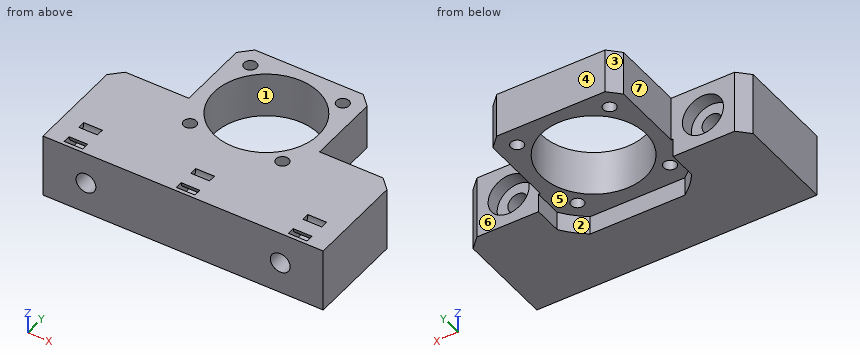
```python
from build123d import *

# Parameters (mm, degrees)
ESQUISSE1_R                                        = 14
ESQUISSE1_R_2                                      = 1.7
BOSS_EXTRU_1_DEPTH                                 = 17
BOSS_EXTRU_2_START                                 = -17
ESQUISSE2_R                                        = 1.7
ESQUISSE2_R_2                                      = 14
BOSS_EXTRU_2_DEPTH                                 = 17
CHAMBRAGE_POUR_VIS_T_TE_RONDE_BOMB_E_M_D           = 5.3
CHAMBRAGE_POUR_VIS_T_TE_RONDE_BOMB_E_M_DEPTH       = 35
CHAMBRAGE_POUR_VIS_T_TE_RONDE_BOMB_E_M_CBORE_D     = 11
CHAMBRAGE_POUR_VIS_T_TE_RONDE_BOMB_E_M_CBORE_DEPTH = 3.7
CHAMBRAGE_POUR_VIS_T_TE_RONDE_BOMB_E_M_TIP         = 1.59228064
ESQUISSE7_W                                        = 5
ESQUISSE7_H                                        = 2
ENL_V_MAT_EXTRU_1_DEPTH                            = 5
ENL_V_MAT_EXTRU_2_DEPTH                            = 5


with BuildPart() as part:
    # Esquisse1 → Boss.-Extru.1 (new body)
    with BuildSketch(Plane.XY):
        with BuildLine():
            Line((12.489995997, 17.5), (-12.489995997, 17.5))
            ThreePointArc((-12.489995997, 17.5), (-15.202795796, 15.202795796), (-17.5, 12.489995997))
            Line((-17.5, 12.489995997), (-17.5, -12.489995997))
            ThreePointArc((-17.5, -12.489995997), (-15.202795796, -15.202795796), (-12.489995997, -17.5))
            Line((-12.489995997, -17.5), (12.489995997, -17.5))
            ThreePointArc((12.489995997, -17.5), (15.202795796, -15.202795796), (17.5, -12.489995997))
            Line((17.5, -12.489995997), (17.5, 12.489995997))
            ThreePointArc((17.5, 12.489995997), (15.202795796, 15.202795796), (12.489995997, 17.5))
        make_face()
        Circle(ESQUISSE1_R, mode=Mode.SUBTRACT)
        with Locations((-12.374368671, -12.374368671)):
            Circle(ESQUISSE1_R_2, mode=Mode.SUBTRACT)
        with Locations((12.374368671, -12.374368671)):
            Circle(ESQUISSE1_R_2, mode=Mode.SUBTRACT)
        with Locations((12.374368671, 12.374368671)):
            Circle(ESQUISSE1_R_2, mode=Mode.SUBTRACT)
        with Locations((-12.374368671, 12.374368671)):
            Circle(ESQUISSE1_R_2, mode=Mode.SUBTRACT)
    extrude(amount=BOSS_EXTRU_1_DEPTH)

    # Esquisse2 → Boss.-Extru.2 (add)
    with BuildSketch(Plane.XY.offset(17).offset(BOSS_EXTRU_2_START)):
        Polygon((-12.489995997, 17.5), (-14.5, 17.5), (-17.5, 14.5), (-17.5, -5), (-34.5, -5), (-37.5, -8), (-37.5, -34.15), (37.5, -34.15), (37.5, -8), (34.5, -5), (17.5, -5), (17.5, 14.5), (14.5, 17.5), align=None)
        with Locations((12.374368671, 12.374368671)):
            Circle(ESQUISSE2_R, mode=Mode.SUBTRACT)
        with Locations((12.374368671, -12.374368671)):
            Circle(ESQUISSE2_R, mode=Mode.SUBTRACT)
        with Locations((-12.374368671, -12.374368671)):
            Circle(ESQUISSE2_R, mode=Mode.SUBTRACT)
        with Locations((-12.374368671, 12.374368671)):
            Circle(ESQUISSE2_R, mode=Mode.SUBTRACT)
        Circle(ESQUISSE2_R_2, mode=Mode.SUBTRACT)
    extrude(amount=BOSS_EXTRU_2_DEPTH)

    # Chambrage pour vis à tête ronde bombée M51
    with Locations(Plane(origin=(0, -5, 0), x_dir=(1, 0, 0), z_dir=(0, 1, 0))):
        with Locations((-26, -8.5), (26, -8.5)):
            CounterBoreHole(CHAMBRAGE_POUR_VIS_T_TE_RONDE_BOMB_E_M_D / 2, CHAMBRAGE_POUR_VIS_T_TE_RONDE_BOMB_E_M_CBORE_D / 2, CHAMBRAGE_POUR_VIS_T_TE_RONDE_BOMB_E_M_CBORE_DEPTH, depth=CHAMBRAGE_POUR_VIS_T_TE_RONDE_BOMB_E_M_DEPTH)
            with Locations((0, 0, -(CHAMBRAGE_POUR_VIS_T_TE_RONDE_BOMB_E_M_DEPTH + CHAMBRAGE_POUR_VIS_T_TE_RONDE_BOMB_E_M_TIP / 2))):  # 118° drill point
                Cone(0, CHAMBRAGE_POUR_VIS_T_TE_RONDE_BOMB_E_M_D / 2, CHAMBRAGE_POUR_VIS_T_TE_RONDE_BOMB_E_M_TIP, mode=Mode.SUBTRACT)

    # Esquisse7 → Enlèvement de matière-Révolution1 (revolve, cut)
    with BuildSketch(Plane.XY.offset(17)):
        with Locations((0, -26.15)):
            Rectangle(ESQUISSE7_W, ESQUISSE7_H)
        with Locations((-30, -26.15)):
            Rectangle(ESQUISSE7_W, ESQUISSE7_H)
        with Locations((30, -26.15)):
            Rectangle(ESQUISSE7_W, ESQUISSE7_H)
    revolve(axis=Axis((-37.5, -29.15, 17), (1, 0, 0)), mode=Mode.SUBTRACT)

    # Esquisse8 → Enlèv. mat.-Extru.1 (cut)
    with BuildSketch(Plane(origin=(0, 0, 0), x_dir=(-1, 0, 0), z_dir=(0, 0, -1))):
        with BuildLine():
            Line((-12.489995997, 17.5), (-14.5, 17.5))
            Line((-14.5, 17.5), (-17.5, 14.5))
            Line((-17.5, 14.5), (-17.5, 12.489995997))
            Line((-17.5, 12.489995997), (-17.5, -12.489995997))
            ThreePointArc((-17.5, -12.489995997), (-15.202795796, -15.202795796), (-12.489995997, -17.5))
            Line((-12.489995997, -17.5), (12.489995997, -17.5))
            ThreePointArc((12.489995997, -17.5), (15.202795796, -15.202795796), (17.5, -12.489995997))
            Line((17.5, -12.489995997), (17.5, 12.489995997))
            Line((17.5, 12.489995997), (17.5, 14.5))
            Line((17.5, 14.5), (14.5, 17.5))
            Line((14.5, 17.5), (12.489995997, 17.5))
            Line((12.489995997, 17.5), (-12.489995997, 17.5))
        make_face()
    extrude(amount=-ENL_V_MAT_EXTRU_1_DEPTH, mode=Mode.SUBTRACT)

    # Esquisse9 → Enlèv. mat.-Extru.2 (cut)
    with BuildSketch(Plane(origin=(0, 0, 0), x_dir=(-1, 0, 0), z_dir=(0, 0, -1))):
        with BuildLine():
            Line((-18, -4.5), (-18, -12.649110641))
            ThreePointArc((-18, -12.649110641), (-15.556349186, -15.556349186), (-12.649110641, -18))
            Line((-12.649110641, -18), (12.649110641, -18))
            ThreePointArc((12.649110641, -18), (15.556349186, -15.556349186), (18, -12.649110641))
            Line((18, -12.649110641), (18, -4.5))
            Line((18, -4.5), (-18, -4.5))
        make_face()
        with BuildLine():
            Line((17.5, -12.489995997), (17.5, -5))
            Line((17.5, -5), (-17.5, -5))
            Line((-17.5, -5), (-17.5, -12.489995997))
            ThreePointArc((-17.5, -12.489995997), (-15.202795796, -15.202795796), (-12.489995997, -17.5))
            Line((-12.489995997, -17.5), (12.489995997, -17.5))
            ThreePointArc((12.489995997, -17.5), (15.202795796, -15.202795796), (17.5, -12.489995997))
        make_face(mode=Mode.SUBTRACT)
    extrude(amount=-ENL_V_MAT_EXTRU_2_DEPTH, mode=Mode.SUBTRACT)


solid = part.part
```
Verification items for the finished model (mm, model axes). Face numbers are marked on the shaded views. A direction names the side the tool comes from. Give positions to 0.01 mm unless a question says otherwise; leave off trailing zeros. Order: outer loops, then holes, each group sorted by start corner. A loop starts at its lowest first (then second) coordinate and runs counter-clockwise, first axis right, second up. Notation, with made-up numbers: M 16,9 L 48,9 A23 ccw 48,30 Z; hole C 15,83 d4. An arc over 180 degrees is marked long. Return JSON: item names as keys, results as strings. Group by question number.
1) Section check D-D on x = 0. Record the cut outline in (y, z).
2) Section check B-B on x = -26. Record the cut outline in (y, z).
3) Mould release check, pull along X, two halves, no side actions. Record for the marked faces 1, 2, 3 and 4: pulls with the +X half, pulls with the -X half, needs draft (parallel to the pull), parting line crosses it, or undercut.
4) Section check C-C on z = 9.25. Give the number of separate pieces and of enclosed holes in the cut face, and give its area (3 significant figures).
5) Scan lines: line 1 (X direction, y = -12.5, z = 2); line 2 (Z direction, x = -26, y = -17); line 3 (X direction, y = 6, z = 12). Record each from-to range of solid material in increasing order.
6) Go/stop test with flat-tipped pins: pin 1 Ø3 at (x, y) = (-12.37, -12.37) entering from -Z; pin 2 Ø4.5 at (x, y) = (12.37, 12.37) entering from -Z; pin 3 Ø4 at (y, z) = (3.5, 13.5) entering from +X. Record where each tip stops, or that it passes through.
7) Access from +Z, -Z, +X, -X, +Y, -Y to the whole of each face (thin tool, end or side, straight path). Record for the marked faces 5, 6 and 7.
8) Section check A-A on y = 0. Record the cut outline in (x, z).
Answer block:
{
 "1": {"outline": "M -34.15,0 L -18,0 L -18,5 L -14,5 L -14,17 L -25.15,17 A4 cw -33.15,17 L -34.15,17 Z; M -31.15,17 A2 ccw -27.15,17 Z; M 14,5 L 17.5,5 L 17.5,17 L 14,17 Z"},
 "2": {"outline": "M -34.15,0 L -5,0 L -5,3 L -8.7,3 L -8.7,5.85 L -34.15,5.85 Z; M -34.15,11.15 L -8.7,11.15 L -8.7,14 L -5,14 L -5,17 L -34.15,17 Z"},
 "3": {"face 1": "undercut", "face 2": "undercut", "face 3": "pulls with the -X half", "face 4": "needs draft"},
 "4": {"separate pieces": "3", "enclosed holes": "5", "area": "1,960 mm^2"},
 "5": {"line 1": "x = -37.5 to -18, 18 to 37.5", "line 2": "z = 0 to 5.85, 11.15 to 17", "line 3": "x = -17.5 to -12.65, 12.65 to 17.5"},
 "6": {"pin 1": "passes through", "pin 2": "stops at z = 5", "pin 3": "stops at x = 17.5"},
 "7": {"face 5": "-Z, +Y", "face 6": "+Z, -Z, +X, +Y", "face 7": "+Z, -Z, -X, +Y"},
 "8": {"outline": "M -17.5,5 L -14,5 L -14,17 L -17.5,17 Z; M 14,5 L 17.5,5 L 17.5,17 L 14,17 Z"}
}
